Can you work these out from the drawing? Everything is in mm from the part's minimum corner. A direction names the side the tool comes from. Round coordinates to 2 decimals unless told otherwise and drop trailing zeros. Write each loop counter-clockwise with the first axis right and the second up, starting at its lowest first coordinate (ties: lowest second). Pieces come first, ordered by that corner, then holes.
Q1. We'd pull the mould along Z, two halves only. Please class the marked faces 1, 2 and 3: +Z half, -Z half, draft (parallel to the pull), parting line (faces both ways), or undercut.
Q2. If we section it at C-C (z = 23): Please give me the cut outline in (x, y), plus the area to 3 significant figures.
Q3. If we section it at A-A (y = 7.5): Please give me the cut outline in (x, z), plus the area to 3 significant figures.
Q4. If we section it at B-B (x = 86): Please give me the cut outline in (y, z), plus the area to 3 significant figures.
Q5. I'm going to push a flat-ended pin straight in: pin 1 Ø5 at (x, y) = (143, 6) entering from +Z. Where does the tip first touch, or does it pass through?
Q6. For the marked faces 4, 5 and 6, which set-ups out of +Z, -Z, +X, -X, +Y, -Y let a thin tool reach every point of the face, with its end or its side?
Q7. If we section it at D-D (y = 1.5): Please give me the cut outline in (x, z), plus the area to 3 significant figures.
Q8. Please list where these lines run through material, in increasing order: line 1 along X through (y, z) = (1.5, 32); line 2 along Z through (x, y) = (7.5, 9); line 3 along Z through (x, y) = (37, 0.75).
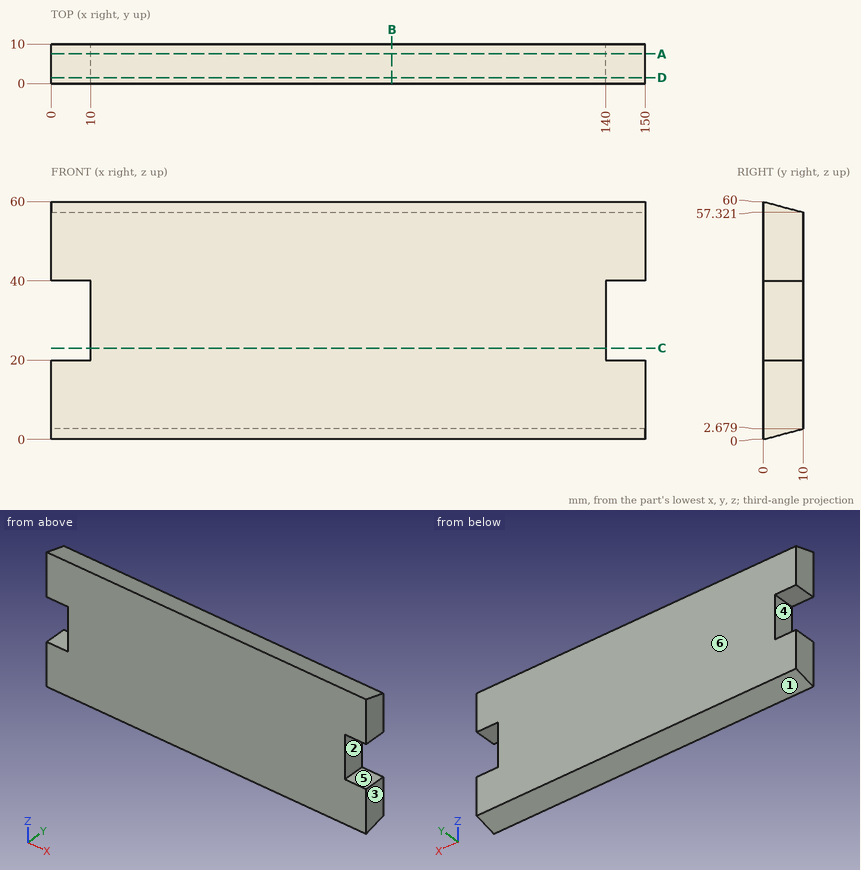
A:
1. face 1: -Z half
1. face 2: undercut
1. face 3: draft
2. outline: (10, 0) - (140, 0) - (140, 10) - (10, 10) - close
2. area: 1,300 mm2
3. outline: (0, 2.01) - (150, 2.01) - (150, 20) - (140, 20) - (140, 40) - (150, 40) - (150, 57.99) - (0, 57.99) - (0, 40) - (10, 40) - (10, 20) - (0, 20) - close
3. area: 8,000 mm2
4. outline: (0, 0) - (10, 2.68) - (10, 57.32) - (0, 60) - close
4. area: 573 mm2
5. pin 1: stops at z = 59.06
6. face 4: -X, +Y, -Y
6. face 5: +X, +Y, -Y
6. face 6: +Z, -Z, +X, -X, +Y
7. outline: (0, 0.4) - (150, 0.4) - (150, 20) - (140, 20) - (140, 40) - (150, 40) - (150, 59.6) - (0, 59.6) - (0, 40) - (10, 40) - (10, 20) - (0, 20) - close
7. area: 8,480 mm2
8. line 1: x = 10 to 140
8. line 2: z = 2.41 to 20, 40 to 57.59
8. line 3: z = 0.2 to 59.8
